The listing builds one solid part. Answer for the finished solid, in the listing's coordinates (mm). Face numbers are marked on the shaded views. A direction names the side the tool comes from. Give positions to 0.01 mm unless a question says otherwise; leave off trailing zeros. Order: outer loops, then holes, each group sorted by start corner. A loop starts at its lowest first (then second) coordinate and runs counter-clockwise, first axis right, second up.
```python
from build123d import *

# Parameters (mm, degrees)
ESQUISSE1_R        = 1.6
BOSS_EXTRU_1_DEPTH = 5


with BuildPart() as part:
    # Esquisse1 → Boss.-Extru.1 (new body)
    with BuildSketch(Plane.XY):
        with BuildLine():
            Line((22.327201908, 31.379603837), (39.110435041, 30.51970557))
            add(Edge.make_bspline(
                [(39.110435041, 30.51970557), (36.47036177, 35.234015671), (31.363758289, 38.634202101), (25.860213157, 38.692785858)],
                knots=[0, 0, 0, 0, 1, 1, 1, 1], degree=3))
            ThreePointArc((25.860213157, 38.692785858), (25.667702993, 38.985657248), (25.860213157, 39.278528639))
            add(Edge.make_bspline(
                [(40.257442964, 30.322056107), (37.254594876, 35.338660309), (31.834783082, 39.118012576), (25.860213157, 39.278528639)],
                knots=[0, 0, 0, 0, 1, 1, 1, 1], degree=3))
            ThreePointArc((40.257442964, 30.322056107), (42.530790825, 28.735523525), (44.029353415, 26.403248607))
            ThreePointArc((44.029353415, 26.403248607), (44.727102443, 25.92851016), (45.42485147, 26.403248607))
            Line((45.42485147, 26.403248607), (47.257362462, 27.428768466))
            Line((47.257362462, 27.428768466), (48.294348688, 26.259658274))
            Line((48.294348688, 26.259658274), (47.257362462, 23.11213505))
            Line((47.257362462, 23.11213505), (46.726853729, 20.169285321))
            ThreePointArc((46.726853729, 20.169285321), (40.667605427, 11.913133381), (43.612357696, 2.104618258))
            add(Edge.make_bspline(
                [(42.15327541, 1.306168032), (43.216115527, 1.058074746), (43.612357696, 2.104618258)],
                knots=[0, 0, 0, 1, 1, 1], degree=2))
            ThreePointArc((42.15327541, 1.306168032), (36.433188896, 10.069245024), (38.395197552, 20.348419608))
            Line((38.395197552, 20.348419608), (37.901995747, 23.976769729))
            Line((37.901995747, 23.976769729), (34.777422909, 24.385367715))
            Line((34.777422909, 24.385367715), (34.63683293, 26.004711162))
            add(Edge.make_bspline(
                [(34.63683293, 26.004711162), (31.667222126, 24.941467321), (27.310515623, 23.524901716), (23.172641891, 19.922056798), (21.279549959, 20.917906985)],
                knots=[0, 0, 0, 0, 0.624834994, 1, 1, 1, 1], degree=3))
            ThreePointArc((21.279549959, 20.917906985), (21.246108661, 21.381188034), (21.68443358, 21.534872503))
            add(Edge.make_bspline(
                [(34.253498198, 26.678639313), (31.663787476, 25.192133844), (27.282995796, 24.602462594), (23.471926653, 20.784486953), (21.68443358, 21.534872503)],
                knots=[0, 0, 0, 0, 0.618454585, 1, 1, 1, 1], degree=3))
            Line((34.253498198, 26.678639313), (18.193151692, 29.841352594))
            ThreePointArc((18.193151692, 29.841352594), (19.619419184, 32.332514308), (22.327201908, 31.379603837))
        make_face()
        with Locations((40.257442964, 27.673893027)):
            Circle(ESQUISSE1_R, mode=Mode.SUBTRACT)
    extrude(amount=BOSS_EXTRU_1_DEPTH)


solid = part.part
```
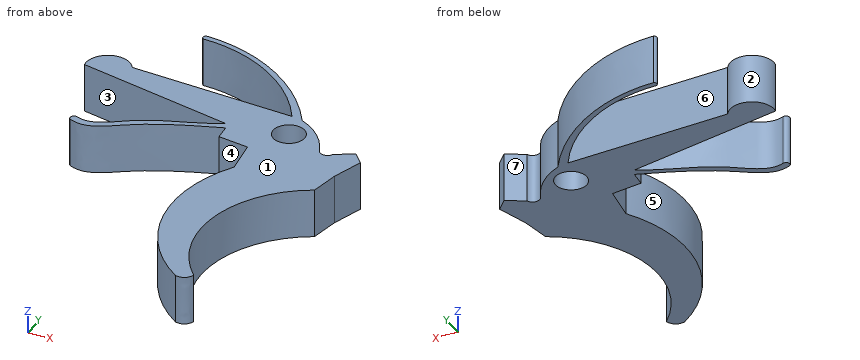
1) A tool of negligible diameter and unlimited length cuts with its end or side. For the marked faces 5, 6 and 7, from which of +Z, -Z, +X, -X, +Y, -Y can it reach the whole face along a straight path? Write none if from no direction.
Geometry says:
face 5: +Z, -Z, -X
face 6: +Z, -Z
face 7: +Z, -Z, +Y
2) Given P1, Ø3, axis at y = 8, z = 1, coming from the +X side; P2, Ø1.5, axis at x = 39.5, z = 2.5, coming from the -Y side; P3, Ø2, axis at y = 29, z = 3, coming from the -X side; P4, Ø3, axis at x = 40.26, y = 27.67, coming from the +Z side, each flat-ended and moving along its own axis, determine where each tip first touches the part or whether it passes through.
Geometry says:
P1: stops at x = 41.04
P2: stops at y = 2.9
P3: stops at x = 18.17
P4: passes through
3) Straight lines are drawn through the part: probe 1 along Y at (x, z) = (37.5, 1.1); probe 2 along Y at (x, z) = (33, 0.3); probe 3 along Y at (x, z) = (23, 1.5). For each, find the intervals that lie inside material, in ascending order.
Geometry says:
probe 1: y = 6.82 to 18.73, 24.03 to 30.6, 32.87 to 33.9
probe 2: y = 25.42 to 26.04, 26.93 to 30.83, 36.69 to 37.31
probe 3: y = 20.6 to 21.35, 28.89 to 31.35
4) Find section B-B (x = 46). Write down the section's boundary in (y, z).
Geometry says:
outline: (19.76, 0) - (26.73, 0) - (26.73, 5) - (19.76, 5) - close
5) For a pull along X with two mould halves and no side action, classify the marked faces 1, 2, 3 and 4 as +X half, -X half, draft (parallel to the pull), parting line (faces both ways), or undercut.
Geometry says:
face 1: draft
face 2: undercut
face 3: -X half
face 4: undercut
6) Find section C-C (y = 13). Write down the section's boundary in (x, z), then the cut area to 3 significant figures.
Geometry says:
outline: (36.17, 0) - (40.91, 0) - (40.91, 5) - (36.17, 5) - close
area: 23.7 mm2
7) Find section A-A (x = 33.5). Count the separate pieces of the cut face and the enclosed holes in it, then the cut area to 3 significant figures.
Geometry says:
separate pieces: 3
enclosed holes: 0
area: 26.5 mm2
